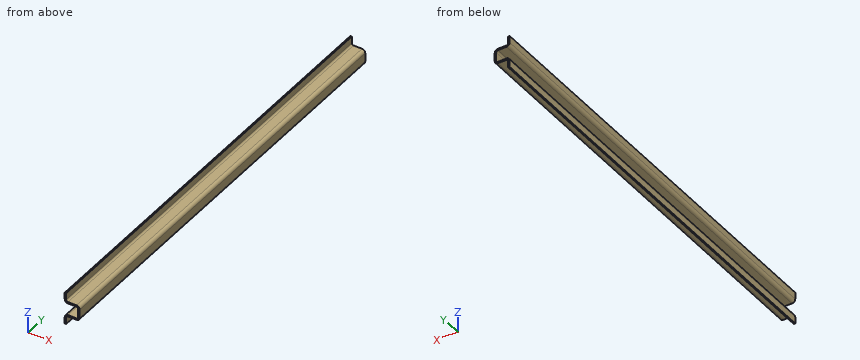
from build123d import *

# Parameters (mm, degrees)
SKETCH2_W                      = 19.05
SKETCH2_H                      = 553.466
BASE_FLANGE1_DEPTH             = 1.89738
EDGE_FLANGE1_STRIP_W           = 11.90752
EDGE_FLANGE1_STRIP_H           = 1.89738
EDGE_FLANGE1_STRIP_CUT_DEPTH   = 553.466
EDGE_FLANGE1_STRIP_2_W         = 11.90752
EDGE_FLANGE1_STRIP_2_H         = 1.89738
EDGE_FLANGE1_STRIP_CUT_2_DEPTH = 553.466
EDGE_FLANGE1_DEPTH             = 553.466
EDGE_FLANGE1_BEND_DEPTH        = 553.466
EDGE_FLANGE2_STRIP_W           = 11.90752
EDGE_FLANGE2_STRIP_H           = 1.89738
EDGE_FLANGE2_STRIP_CUT_DEPTH   = 553.466
EDGE_FLANGE2_STRIP_2_W         = 11.90752
EDGE_FLANGE2_STRIP_2_H         = 1.89738
EDGE_FLANGE2_STRIP_CUT_2_DEPTH = 553.466
EDGE_FLANGE2_DEPTH             = 553.466
EDGE_FLANGE2_BEND_DEPTH        = 553.466


# Sheet-metal steps are written as plain solids
with BuildPart() as part:
    # Sketch2 → Base-Flange1 (new body)
    with BuildSketch(Plane(origin=(0, 0, 0), x_dir=(0, 0, -1), z_dir=(1, 0, 0))):
        Rectangle(SKETCH2_W, SKETCH2_H)
    extrude(amount=-BASE_FLANGE1_DEPTH)

    # Edge-Flange1 strip (across the edge) → Edge-Flange1 strip cut (cut)
    with BuildSketch(Plane(origin=(-1.89738, -276.733, 9.525), x_dir=(0, 0, -1), z_dir=(0, 1, 0))):
        with Locations((-1.89738, -0.94869)):
            Rectangle(EDGE_FLANGE1_STRIP_W, EDGE_FLANGE1_STRIP_H)
    extrude(amount=EDGE_FLANGE1_STRIP_CUT_DEPTH, mode=Mode.SUBTRACT)

    # Edge-Flange1 strip 2 (across the edge) → Edge-Flange1 strip cut 2 (cut)
    with BuildSketch(Plane(origin=(-1.89738, 276.733, -9.525), x_dir=(0, 0, 1), z_dir=(0, -1, 0))):
        with Locations((-1.89738, -0.94869)):
            Rectangle(EDGE_FLANGE1_STRIP_2_W, EDGE_FLANGE1_STRIP_2_H)
    extrude(amount=EDGE_FLANGE1_STRIP_CUT_2_DEPTH, mode=Mode.SUBTRACT)

    # Edge-Flange1 section (across the edge) → Edge-Flange1 (add)
    with BuildSketch(Plane(origin=(-1.89738, -276.733, 9.525), x_dir=(0, 0, -1), z_dir=(0, 1, 0))):
        with BuildLine():
            Line((0, 2.159), (0, 17.15262))
            Line((0, 17.15262), (1.89738, 17.15262))
            Line((1.89738, 17.15262), (1.89738, 2.159))
            ThreePointArc((1.89738, 2.159), (2.529736459, 0.632356459), (4.05638, 0))
            Line((4.05638, 0), (4.05638, -1.89738))
            ThreePointArc((4.05638, -1.89738), (1.188086195, -0.709293805), (0, 2.159))
        make_face()
    extrude(amount=EDGE_FLANGE1_DEPTH)

    # Edge-Flange1 section 2 (across the edge) → Edge-Flange1 bend (add)
    with BuildSketch(Plane(origin=(-1.89738, 276.733, -9.525), x_dir=(0, 0, 1), z_dir=(0, -1, 0))):
        with BuildLine():
            Line((0, 2.159), (0, 17.15262))
            Line((0, 17.15262), (1.89738, 17.15262))
            Line((1.89738, 17.15262), (1.89738, 2.159))
            ThreePointArc((1.89738, 2.159), (2.529736459, 0.632356459), (4.05638, 0))
            Line((4.05638, 0), (4.05638, -1.89738))
            ThreePointArc((4.05638, -1.89738), (1.188086195, -0.709293805), (0, 2.159))
        make_face()
    extrude(amount=EDGE_FLANGE1_BEND_DEPTH)

    # Edge-Flange2 strip (across the edge) → Edge-Flange2 strip cut (cut)
    with BuildSketch(Plane(origin=(-19.05, -276.733, -9.525), x_dir=(1, 0, 0), z_dir=(0, 1, 0))):
        with Locations((-1.89738, -0.94869)):
            Rectangle(EDGE_FLANGE2_STRIP_W, EDGE_FLANGE2_STRIP_H)
    extrude(amount=EDGE_FLANGE2_STRIP_CUT_DEPTH, mode=Mode.SUBTRACT)

    # Edge-Flange2 strip 2 (across the edge) → Edge-Flange2 strip cut 2 (cut)
    with BuildSketch(Plane(origin=(-19.05, 276.733, 9.525), x_dir=(1, 0, 0), z_dir=(0, -1, 0))):
        with Locations((-1.89738, -0.94869)):
            Rectangle(EDGE_FLANGE2_STRIP_2_W, EDGE_FLANGE2_STRIP_2_H)
    extrude(amount=EDGE_FLANGE2_STRIP_CUT_2_DEPTH, mode=Mode.SUBTRACT)

    # Edge-Flange2 section (across the edge) → Edge-Flange2 (add)
    with BuildSketch(Plane(origin=(-19.05, -276.733, -9.525), x_dir=(1, 0, 0), z_dir=(0, 1, 0))):
        with BuildLine():
            Line((0, 2.159), (0, 10.80262))
            Line((0, 10.80262), (1.89738, 10.80262))
            Line((1.89738, 10.80262), (1.89738, 2.159))
            ThreePointArc((1.89738, 2.159), (2.529736459, 0.632356459), (4.05638, 0))
            Line((4.05638, 0), (4.05638, -1.89738))
            ThreePointArc((4.05638, -1.89738), (1.188086195, -0.709293805), (0, 2.159))
        make_face()
    extrude(amount=EDGE_FLANGE2_DEPTH)

    # Edge-Flange2 section 2 (across the edge) → Edge-Flange2 bend (add)
    with BuildSketch(Plane(origin=(-19.05, 276.733, 9.525), x_dir=(1, 0, 0), z_dir=(0, -1, 0))):
        with BuildLine():
            Line((0, 2.159), (0, 10.80262))
            Line((0, 10.80262), (1.89738, 10.80262))
            Line((1.89738, 10.80262), (1.89738, 2.159))
            ThreePointArc((1.89738, 2.159), (2.529736459, 0.632356459), (4.05638, 0))
            Line((4.05638, 0), (4.05638, -1.89738))
            ThreePointArc((4.05638, -1.89738), (1.188086195, -0.709293805), (0, 2.159))
        make_face()
    extrude(amount=EDGE_FLANGE2_BEND_DEPTH)


solid = part.part
Geometry check sheet. Reference: the model listing, model coordinates, mm. Give positions to 0.01 mm unless a question says otherwise; leave off trailing zeros. Order: outer loops, then holes, each group sorted by start corner. A loop starts at its lowest first (then second) coordinate and runs counter-clockwise, first axis right, second up.
1) Cross-section at A-A (x = -7). Record the boundary of the cut face in (y, z) (3 decimals), then the cut area to 3 significant figures.
Results are:
outline: (-276.733, -9.525) - (276.733, -9.525) - (276.733, -7.628) - (-276.733, -7.628) - close; (-276.733, 7.628) - (276.733, 7.628) - (276.733, 9.525) - (-276.733, 9.525) - close
area: 2,100 mm2
2) Gauge pin test, flat ends, axial feed: pin 1 (8.5 mm diameter, centred on y = -136, z = -1, fed in from -X); pin 2 (3.5 mm diameter, centred on x = -10, y = 121.5, fed in from -Z) (3 decimals); pin 3 (10 mm diameter, centred on x = -8, y = 2, fed in from +Z) (3 decimals). Record the tip position at first contact, or that the pin passes through.
Results are:
pin 1: stops at x = -1.9
pin 2: stops at z = -9.525
pin 3: stops at z = 9.525
3) Cross-section at C-C (z = 1). Record the boundary of the cut face in (x, y).
Results are:
outline: (-1.9, -276.73) - (0, -276.73) - (0, 276.73) - (-1.9, 276.73) - close
4) Cross-section at B-B (y = 154). Record the boundary of the cut face in (x, z) (3 decimals), then the cut area to 3 significant figures.
Results are:
outline: (-19.05, -20.328) - (-17.153, -20.328) - (-17.153, -11.684) arc R2.159 cw to (-14.994, -9.525) - (-4.056, -9.525) arc R4.056 ccw to (0, -5.469) - (0, 5.469) arc R4.056 ccw to (-4.056, 9.525) - (-14.994, 9.525) arc R2.159 cw to (-17.153, 11.684) - (-17.153, 20.328) - (-19.05, 20.328) - (-19.05, 11.684) arc R4.056 ccw to (-14.994, 7.628) - (-4.056, 7.628) arc R2.159 cw to (-1.897, 5.469) - (-1.897, -5.469) arc R2.159 cw to (-4.056, -7.628) - (-14.994, -7.628) arc R4.056 ccw to (-19.05, -11.684) - close
area: 132 mm2
5) Material ranges on probe 1 along Z at (x, y) = (-14.5, 80) (3 decimals); probe 2 along X at (y, z) = (238, 2); probe 3 along X at (y, z) = (7.5, 14), recorded low to high.
Results are:
probe 1: z = -9.525 to -7.628, 7.628 to 9.525
probe 2: x = -1.9 to 0
probe 3: x = -19.05 to -17.15
